Verification items for the finished model (mm, model axes). Give positions to 0.01 mm unless a question says otherwise; leave off trailing zeros. Write each loop counter-clockwise with the first axis right and the second up, starting at its lowest first coordinate (ties: lowest second). Pieces come first, ordered by that corner, then holes. Notation, with made-up numbers: M 39.25,50 L 85.25,50 A35 cw 85.25,89 Z; hole C 1.5,-39.5 d8. An arc over 180 degrees is marked long. Answer as a JSON object with one key per item and string values.
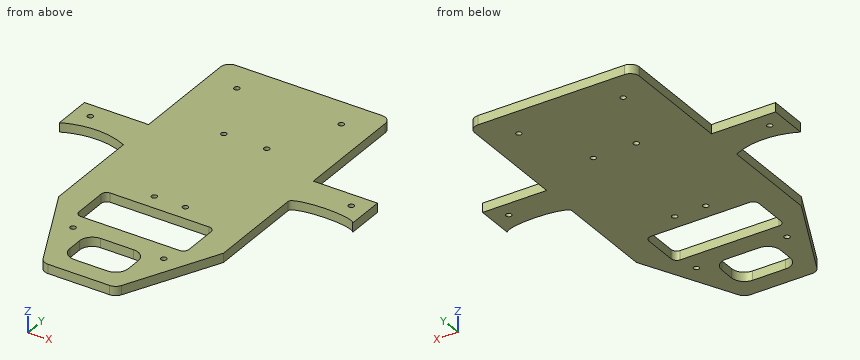
```python
from build123d import *

# Parameters (mm, degrees)
BOSS_EXTRUDE1_DEPTH = 5
SKETCH3_R           = 1.5
CUT_EXTRUDE1_DEPTH  = 146.976025571
CUT_EXTRUDE2_DEPTH  = 146.976025571
SKETCH5_R           = 1.5
CUT_EXTRUDE3_DEPTH  = 146.976025571
CUT_EXTRUDE4_DEPTH  = 146.976025571
SKETCH7_R           = 1.5
CUT_EXTRUDE5_DEPTH  = 146.976025571


with BuildPart() as part:
    # Sketch2 → Boss-Extrude1 (new body)
    with BuildSketch(Plane.XY):
        with BuildLine():
            Line((-45, -70), (-21.362272993, -119.166472174))
            ThreePointArc((-21.362272993, -119.166472174), (-19.517555453, -121.23275093), (-16.85601087, -122))
            Line((-16.85601087, -122), (16.85601087, -122))
            ThreePointArc((16.85601087, -122), (19.517555453, -121.23275093), (21.362272993, -119.166472174))
            Line((21.362272993, -119.166472174), (45, -70))
            Line((45, -70), (45, -16))
            add(Edge.make_bspline(
                [(80, -16), (80, -12), (62.5, -12), (45, -12), (45, -16)],
                knots=[3.141592654, 3.141592654, 3.141592654, 4.71238898, 4.71238898, 6.283185307, 6.283185307, 6.283185307], degree=2, weights=[1, 0.707106781, 1, 0.707106781, 1]))
            Line((80, -16), (80, 5))
            Line((80, 5), (45, 5))
            Line((45, 5), (45, 65))
            ThreePointArc((45, 65), (43.535533906, 68.535533906), (40, 70))
            Line((40, 70), (-40, 70))
            ThreePointArc((-40, 70), (-43.535533906, 68.535533906), (-45, 65))
            Line((-45, 65), (-45, 5))
            Line((-45, 5), (-80, 5))
            Line((-80, 5), (-80, -16))
            add(Edge.make_bspline(
                [(-45, -16), (-62.5, -7.544335015), (-80, -16)],
                knots=[3.141592654, 3.141592654, 3.141592654, 4.041796627, 4.041796627, 4.041796627], degree=2, weights=[1, 0.900402737, 1]))
            Line((-45, -16), (-45, -70))
        make_face()
    extrude(amount=BOSS_EXTRUDE1_DEPTH)

    # Sketch3 → Cut-Extrude1 (cut, through all)
    with BuildSketch(Plane.XY.offset(5)):
        with Locations((-71.25, -3.49687094)):
            Circle(SKETCH3_R)
        with Locations((71.25, -3.5)):
            Circle(SKETCH3_R)
    extrude(amount=-CUT_EXTRUDE1_DEPTH, mode=Mode.SUBTRACT)

    # Sketch4 → Cut-Extrude2 (cut, through all)
    with BuildSketch(Plane.XY.offset(5)):
        with BuildLine():
            Line((-9, -90), (9, -90))
            ThreePointArc((9, -90), (13.949747468, -92.050252532), (16, -97))
            Line((16, -97), (16, -105))
            ThreePointArc((16, -105), (13.949747468, -109.949747468), (9, -112))
            Line((9, -112), (-9, -112))
            ThreePointArc((-9, -112), (-13.949747468, -109.949747468), (-16, -105))
            Line((-16, -105), (-16, -97))
            ThreePointArc((-16, -97), (-13.949747468, -92.050252532), (-9, -90))
        make_face()
    extrude(amount=-CUT_EXTRUDE2_DEPTH, mode=Mode.SUBTRACT)

    # Sketch5 → Cut-Extrude3 (cut, through all)
    with BuildSketch(Plane.XY.offset(5)):
        with Locations((11.725, 16.949973779)):
            Circle(SKETCH5_R)
        with Locations((-11.725, 16.949973779)):
            Circle(SKETCH5_R)
    extrude(amount=-CUT_EXTRUDE3_DEPTH, mode=Mode.SUBTRACT)

    # Sketch6 → Cut-Extrude4 (cut, through all)
    with BuildSketch(Plane.XY.offset(5)):
        with BuildLine():
            Line((-27, -54.5), (27, -54.5))
            ThreePointArc((27, -54.5), (29.121320344, -55.378679656), (30, -57.5))
            Line((30, -57.5), (30, -76))
            ThreePointArc((30, -76), (29.121320344, -78.121320344), (27, -79))
            Line((27, -79), (-27, -79))
            ThreePointArc((-27, -79), (-29.121320344, -78.121320344), (-30, -76))
            Line((-30, -76), (-30, -57.5))
            ThreePointArc((-30, -57.5), (-29.121320344, -55.378679656), (-27, -54.5))
        make_face()
    extrude(amount=-CUT_EXTRUDE4_DEPTH, mode=Mode.SUBTRACT)

    # Sketch7 → Cut-Extrude5 (cut, through all)
    with BuildSketch(Plane.XY.offset(5)):
        with Locations((-28.5, 53.5)):
            Circle(SKETCH7_R)
        with Locations((28.5, 53.5)):
            Circle(SKETCH7_R)
        with Locations((-24.769714049, -89)):
            Circle(SKETCH7_R)
        with Locations((24.769714049, -89)):
            Circle(SKETCH7_R)
        with Locations((-8.5, -46)):
            Circle(SKETCH7_R)
        with Locations((8.5, -46)):
            Circle(SKETCH7_R)
    extrude(amount=-CUT_EXTRUDE5_DEPTH, mode=Mode.SUBTRACT)


solid = part.part
```
1) Section check D-D on z = 2. Count the separate pieces of the cut face and the enclosed holes in it, and give its area (3 significant figures).
Completed:
{"separate pieces": "1", "enclosed holes": "12", "area": "15,000 mm2"}
2) Thickness scan on L1, parallel to Y at x = 8.5, z = 1.4; L2, parallel to Y at x = 11, z = 0.8; L3, parallel to Y at x = 17, z = 0.95. Record the ranges inside material, lowest first.
Completed:
{"L1": "y = -122 to -112, -90 to -79, -54.5 to -47.5, -44.5 to 70", "L2": "y = -122 to -111.71, -90.29 to -79, -54.5 to 15.64, 18.26 to 70", "L3": "y = -122 to -79, -54.5 to 70"}
3) Section check C-C on x = -33. Record the boundary of the cut face in (y, z), and give its area (3 significant figures).
Completed:
{"outline": "M -94.96,0 L 70,0 L 70,5 L -94.96,5 Z", "area": "825 mm2"}
4) Section check B-B on y = -74. Record the boundary of the cut face in (x, z).
Completed:
{"outline": "M -43.08,0 L -30,0 L -30,5 L -43.08,5 Z; M 30,0 L 43.08,0 L 43.08,5 L 30,5 Z"}
5) Go/stop test with flat-tipped pins: pin 1 (1.5 mm diameter, centred on x = -54.5, z = 3, fed in from +Y); pin 2 (2.5 mm diameter, centred on y = -68, z = 3, fed in from +X); pin 3 (1 mm diameter, centred on x = -44, z = 2.5, fed in from +Y). Record where each tip stops, or that it passes through.
Completed:
{"pin 1": "stops at y = 5", "pin 2": "stops at x = 45", "pin 3": "stops at y = 68.57"}
6) Section check A-A on x = 4. Record the boundary of the cut face in (y, z).
Completed:
{"outline": "M -122,0 L -112,0 L -112,5 L -122,5 Z; M -90,0 L -79,0 L -79,5 L -90,5 Z; M -54.5,0 L 70,0 L 70,5 L -54.5,5 Z"}
